The model under review builds one solid part; all positions refer to its coordinate system, in mm. A direction names the side the tool comes from. Give positions to 0.01 mm unless a question says otherwise; leave off trailing zeros. Loops run counter-clockwise (first coordinate to the right, second up) from the corner with the lowest first, then second, coordinate; pieces in that order, holes last. Notation, with made-up numbers: M 10.25,-29.75 L 15.25,-29.75 A17 ccw 15.25,-14.75 Z; hole C 77,76 d5. An arc over 180 degrees is marked long. Write item = value, one per line. Start each with the question number.
1. For faces 3 (the face through (-30.208, 1.268, -37.273)), 4 (the face through (-5.1, 13, -55)), 5 (the face through (0, 9.4, 49)), list the 3-axis set-ups (+Z, -Z, +X, -X, +Y, -Y) from which the entire face can be reached by the end or side of a thin tool; tool diameter is ignored.
2. Draft analysis for pull direction X (two halves, no side actions). For faces 1 (the face through (0, 23, -49)), 2 (the face through (-29.372, 1.268, 36.276)), state which applies: pulls with the +X half, pulls with the -X half, needs draft (parallel to the pull), parting line crosses it, or undercut.
3. Wall thickness on line 1 along X through (y, z) = (6.25, -52); line 2 along Z through (x, y) = (-1.5, 14); line 3 along Y through (x, z) = (51, 24): over which ranges is each line inside the solid? List them lowest first. Write a range as from..to.
4. We need section D-D on z = -44. Give the boundary of the cut face in (x, y), then the cut area to 3 significant figures.
5. For pin 1 (1 mm diameter, centred on x = -14.5, y = 9, fed in from -Z); pin 2 (1.7 mm diameter, centred on y = 17.5, z = -55.5, fed in from -X); pin 3 (3 mm diameter, centred on y = 12, z = 52.5, fed in from +X); pin 4 (5.5 mm diameter, centred on x = 33, z = 0, fed in from -Y), all flat-tipped, find the tip position at first contact; note any pin that passes through.
6. We need section C-C on z = -30.5. Give the boundary of the cut face in (x, y), then the cut area to 3 significant figures.
7. We need section A-A on x = -31. Give the boundary of the cut face in (y, z).
from build123d import *

# Parameters (mm, degrees)
SKETCH1_R               = 60
BOSS_EXTRUDE1_DEPTH     = 2.5
SKETCH2_R               = 60
SKETCH2_R_2             = 58
BOSS_EXTRUDE2_DEPTH     = 20.5
SKETCH3_R               = 4.5
SKETCH3_R_2             = 5
CUT_EXTRUDE1_DEPTH      = 88.294043325
SKETCH4_W               = 24
SKETCH4_H               = 8
CUT_EXTRUDE2_DEPTH      = 88.294043325
FILLET1_R               = 1
SKETCH5_R               = 2.1
BOSS_EXTRUDE3_DEPTH     = 20.5
CUT_EXTRUDE3_START      = -3.6
CUT_EXTRUDE3_DEPTH      = 3.6
CUT_EXTRUDE4_REACH      = 138.121
CUT_EXTRUDE4_END_RADIUS = 58


with BuildPart() as part:
    # Sketch1 → Boss-Extrude1 (new body)
    with BuildSketch(Plane(origin=(0, 0, 0), x_dir=(1, 0, 0), z_dir=(0, 1, 0))):
        with Locations(Location((0, 0, 0), (0, 0, 270))):
            Circle(SKETCH1_R)
    extrude(amount=BOSS_EXTRUDE1_DEPTH)

    # Sketch2 → Boss-Extrude2 (add)
    with BuildSketch(Plane(origin=(0, 2.5, 0), x_dir=(1, 0, 0), z_dir=(0, 1, 0))):
        with Locations(Location((0, 0, 0), (0, 0, 270))):
            Circle(SKETCH2_R)
        with Locations(Location((0, 0, 0), (0, 0, 270))):
            Circle(SKETCH2_R_2, mode=Mode.SUBTRACT)
    extrude(amount=BOSS_EXTRUDE2_DEPTH)

    # Sketch3 → Cut-Extrude1 (cut, through all)
    with BuildSketch(Plane(origin=(0, 2.5, 0), x_dir=(1, 0, 0), z_dir=(0, 1, 0))):
        with Locations(Location((33, 0, 0), (0, 0, 270))):
            Circle(SKETCH3_R)
        with Locations(Location((33.587572106, 33.587572106, 0), (0, 0, 270))):
            Circle(SKETCH3_R_2)
        with Locations(Location((33.587572106, -33.587572106, 0), (0, 0, 270))):
            Circle(SKETCH3_R_2)
        with Locations(Location((-33.587572106, -33.587572106, 0), (0, 0, 270))):
            Circle(SKETCH3_R_2)
        with Locations(Location((-33.587572106, 33.587572106, 0), (0, 0, 270))):
            Circle(SKETCH3_R_2)
    extrude(amount=-CUT_EXTRUDE1_DEPTH, mode=Mode.SUBTRACT)

    # Sketch4 → Cut-Extrude2 (cut, through all)
    with BuildSketch(Plane(origin=(0, 2.5, 0), x_dir=(1, 0, 0), z_dir=(0, 1, 0))):
        with Locations((-26, -3)):
            Rectangle(SKETCH4_W, SKETCH4_H)
    extrude(amount=-CUT_EXTRUDE2_DEPTH, mode=Mode.SUBTRACT)

    # Fillet1
    fillet1_edges = [part.edges().sort_by_distance(p)[0] for p in [
        (-38, 1.25, 7),
        (-38, 1.25, -1),
        (-14, 1.25, -1),
        (-14, 1.25, 7),
    ]]
    fillet(fillet1_edges, radius=FILLET1_R)

    # Sketch5 → Boss-Extrude3 (add, through all)
    # profile 1 of 2: a face of its own
    with BuildSketch(Plane(origin=(0, 2.5, 0), x_dir=(1, 0, 0), z_dir=(0, 1, 0))):
        with BuildLine():
            Line((-5.1, 52), (-5.1, 57.775340761))
            ThreePointArc((-5.1, 57.775340761), (0, 58), (5.1, 57.775340761))
            Line((5.1, 57.775340761), (5.1, 52))
            ThreePointArc((5.1, 52), (0, 46.9), (-5.1, 52))
        make_face()
        with Locations(Location((0, 52, 0), (0, 0, 270))):
            Circle(SKETCH5_R, mode=Mode.SUBTRACT)
    # profile 2 of 2: a face of its own
    with BuildSketch(Plane(origin=(0, 2.5, 0), x_dir=(1, 0, 0), z_dir=(0, 1, 0))):
        with BuildLine():
            Line((5.1, -52), (5.1, -57.775340761))
            ThreePointArc((5.1, -57.775340761), (0, -58), (-5.1, -57.775340761))
            Line((-5.1, -57.775340761), (-5.1, -52))
            ThreePointArc((-5.1, -52), (0, -46.9), (5.1, -52))
        make_face()
        with Locations(Location((0, -52, 0), (0, 0, 90))):
            Circle(SKETCH5_R, mode=Mode.SUBTRACT)
    extrude(amount=BOSS_EXTRUDE3_DEPTH)

    # Sketch6 → Cut-Extrude3 (cut)
    with BuildSketch(Plane(origin=(0, 13, 0), x_dir=(1, 0, 0), z_dir=(0, 1, 0)).offset(CUT_EXTRUDE3_START)):
        with BuildLine():
            Line((3.6, 54.078460969), (0, 56.156921938))
            Line((0, 56.156921938), (-3.6, 54.078460969))
            Line((-3.6, 54.078460969), (-3.6, 48.387521626))
            ThreePointArc((-3.6, 48.387521626), (0, 46.9), (3.6, 48.387521626))
            Line((3.6, 48.387521626), (3.6, 54.078460969))
        make_face()
        with BuildLine():
            Line((3.6, -48.387521626), (3.6, -54.078460969))
            Line((3.6, -54.078460969), (0, -56.156921938))
            Line((0, -56.156921938), (-3.6, -54.078460969))
            Line((-3.6, -54.078460969), (-3.6, -48.387521626))
            ThreePointArc((-3.6, -48.387521626), (0, -46.9), (3.6, -48.387521626))
        make_face()
    extrude(amount=CUT_EXTRUDE3_DEPTH, mode=Mode.SUBTRACT)

    # Cut-Extrude4: up to this cylinder (the profile starts outside it)
    cut_extrude4_end = Plane(origin=(0, 16, 0), z_dir=(0, -1, 0)) * Cylinder(CUT_EXTRUDE4_END_RADIUS, 393.242, mode=Mode.PRIVATE)
    # Sketch7 → Cut-Extrude4 (cut, up to the surface)
    with BuildSketch(Plane.ZY.offset(60), mode=Mode.PRIVATE) as cut_extrude4_sk1:
        with BuildLine():
            Line((-5, 19), (5, 19))
            ThreePointArc((5, 19), (8, 16), (5, 13))
            Line((5, 13), (-5, 13))
            ThreePointArc((-5, 13), (-8, 16), (-5, 19))
        make_face()
    cut_extrude4_tool1 = extrude(cut_extrude4_sk1.sketch, amount=-CUT_EXTRUDE4_REACH, mode=Mode.PRIVATE) - cut_extrude4_end
    add(cut_extrude4_tool1.solids().sort_by_distance((-60, 16, 0))[0], mode=Mode.SUBTRACT)


solid = part.part
Final values:
q1.face_3 = +Y, -Y
q1.face_4 = +Y
q1.face_5 = none
q2.face_1 = needs draft
q2.face_2 = undercut
q3.line_1 = -29.93..-25.69, -5.1..-2.1, 2.1..5.1, 25.69..29.93
q3.line_2 = -59.98..-53.47, -50.53..-47.13, 47.13..50.53, 53.47..59.98
q3.line_3 = 0..2.5
q4.outline = M -40.79,0 L 40.79,0 L 40.79,23 L 37.79,23 L 37.79,2.5 L -37.79,2.5 L -37.79,23 L -40.79,23 Z
q4.area = 327 mm²
q5.pin_1 = -58.34
q5.pin_2 = -24.77
q5.pin_3 = 31.61
q5.pin_4 = through
q6.outline = M -51.67,0 L -37.52,0 L -37.52,2.5 L -49.33,2.5 L -49.33,23 L -51.67,23 Z; M -29.65,0 L 29.65,0 L 29.65,2.5 L -29.65,2.5 Z; M 37.52,0 L 51.67,0 L 51.67,23 L 49.33,23 L 49.33,2.5 L 37.52,2.5 Z
q6.area = 315 mm²
q7.outline = M 0,-51.37 L 23,-51.37 L 23,-49.02 L 2.5,-49.02 L 2.5,-37.87 L 0,-37.87 Z; M 0,-29.31 L 2.5,-29.31 L 2.5,-1 L 0,-1 Z; M 0,7 L 2.5,7 L 2.5,29.31 L 0,29.31 Z; M 0,37.87 L 2.5,37.87 L 2.5,49.02 L 23,49.02 L 23,51.37 L 0,51.37 Z
